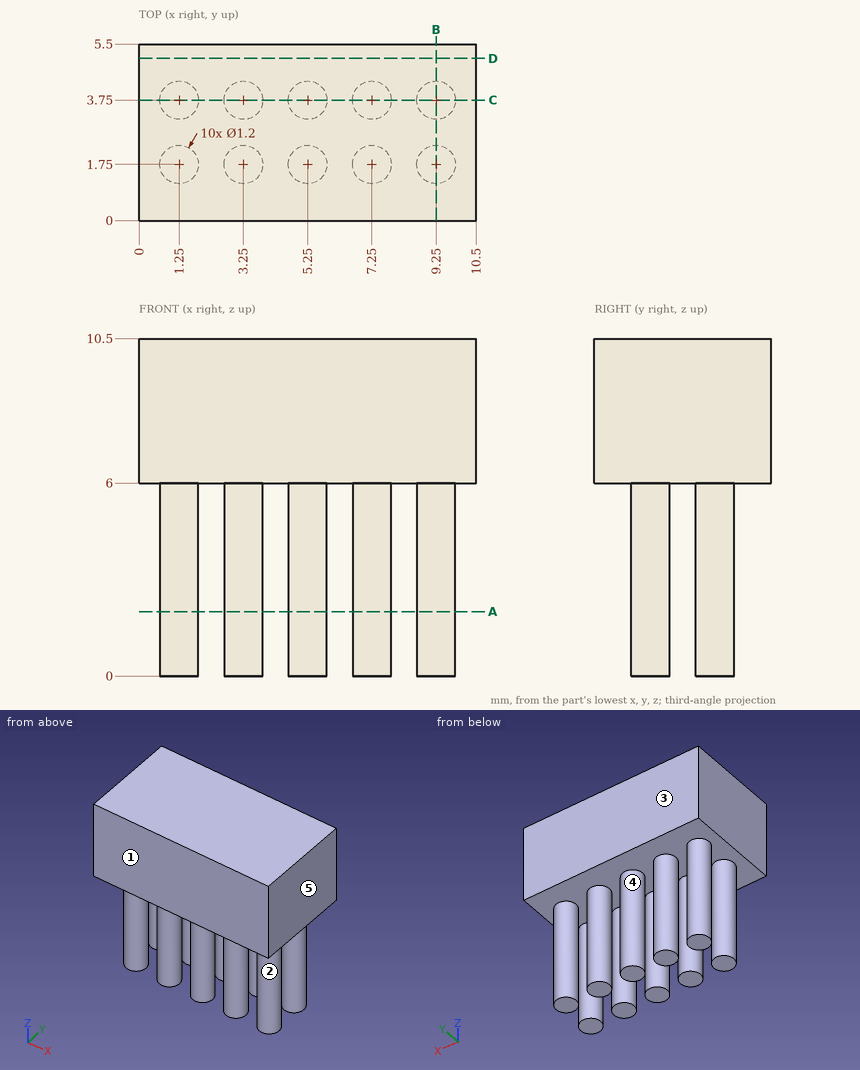
Geometry: see drawing. Coordinates: mm, zero at the bounding-box minimum. A direction names the side the tool comes from. Round coordinates to 2 decimals unless told otherwise and drop trailing zeros. Loops run counter-clockwise (first coordinate to the right, second up) from the corner with the lowest first, then second, coordinate; pieces in that order, holes last. Notation, with made-up numbers: (70, 34) - (79, 34) arc R22 ccw to (79, 58) - close; hole circle Ø8 at (57.5, 71.5). An arc over 180 degrees is marked (long way). One line per item, written item: value. Start each with the question number.
(1) Section B-B, the plane x = 9.25. Return loops of the section in (y, z).
(2) Access query for the marked faces 1 and 2. Directions: +Z, -Z, +X, -X, +Y, -Y. A direction counts if a zero-diameter tool reaches every point of the face in a straight line with its end or side. Return the directions, or none.
(3) Draft query along Y for the marked faces 3, 4 and 5. Return one class per face: +Y half, -Y half, draft (parallel to the pull), parting line (faces both ways), or undercut.
(4) Section A-A, the plane z = 2. Count the separate pieces of the cut face and the enclosed holes in it, plus the area to 3 significant figures.
(5) Section D-D, the plane y = 5.05. Return loops of the section in (x, z).
(6) Section C-C, the plane y = 3.75. Return loops of the section in (x, z), plus the area to 4 significant figures.
(7) Ray query, line 1 (X direction, y = 3.7, z = 2.25); line 2 (Y direction, x = 1.25, z = 3.5); line 3 (Z direction, x = 8.25, y = 2.65). Return the intervals inside material, ascending. Write a range as [from, to].
(8) Contact query for flat-ended pins moving along their axis: P1, Ø2, axis at x = 6.5, z = 2.5, coming from the +Y side; P2, Ø3, axis at y = 3.5, z = 2, coming from the -X side. Output: stop coordinate, or through.
Results below:
1. outline: (0, 6) - (1.15, 6) - (1.15, 0) - (2.35, 0) - (2.35, 6) - (3.15, 6) - (3.15, 0) - (4.35, 0) - (4.35, 6) - (5.5, 6) - (5.5, 10.5) - (0, 10.5) - close
2. face 1: +Z, -Z, +X, -X, -Y
2. face 2: -Z
3. face 3: +Y half
3. face 4: undercut
3. face 5: draft
4. separate pieces: 10
4. enclosed holes: 0
4. area: 11.3 mm^2
5. outline: (0, 6) - (10.5, 6) - (10.5, 10.5) - (0, 10.5) - close
6. outline: (0, 6) - (0.65, 6) - (0.65, 0) - (1.85, 0) - (1.85, 6) - (2.65, 6) - (2.65, 0) - (3.85, 0) - (3.85, 6) - (4.65, 6) - (4.65, 0) - (5.85, 0) - (5.85, 6) - (6.65, 6) - (6.65, 0) - (7.85, 0) - (7.85, 6) - (8.65, 6) - (8.65, 0) - (9.85, 0) - (9.85, 6) - (10.5, 6) - (10.5, 10.5) - (0, 10.5) - close
6. area: 83.25 mm^2
7. line 1: [0.65, 1.85], [2.65, 3.85], [4.65, 5.85], [6.65, 7.85], [8.65, 9.85]
7. line 2: [1.15, 2.35], [3.15, 4.35]
7. line 3: [6, 10.5]
8. P1: y = 4.35
8. P2: x = 0.65
